from build123d import *

# Parameters (mm, degrees)
BOSS_EXTRUDE2_DEPTH         = 23
SHELL1_START                = 5
SHELL1_OUTLINE_W            = 16
SHELL1_OUTLINE_H            = 13
SHELL1_DEPTH                = 15
FILLET1_R                   = 2
FILLET3_R                   = 2
TAP_DRILL_FOR_M4X0_7_TAP1_D = 3.3


# Read off the part's stored shape, not the designer's step: Shell1
with BuildPart() as part:
    # Sketch1 → Boss-Extrude2 (new body)
    with BuildSketch(Plane.XY):
        Polygon((0, 0), (0, 20), (5, 20), (20, 5), (20, 0), align=None)
    extrude(amount=-BOSS_EXTRUDE2_DEPTH)

    # Shell1 outline → Shell1 (cut)
    with BuildSketch(Plane(origin=(0, 0, 0), x_dir=(1, 0, 0), z_dir=(0, 1, 0)).offset(SHELL1_START)):
        with Locations((13, 11.5)):
            Rectangle(SHELL1_OUTLINE_W, SHELL1_OUTLINE_H)
    extrude(amount=SHELL1_DEPTH, mode=Mode.SUBTRACT)

    # Fillet1
    fillet1_edges = [part.edges().sort_by_distance(p)[0] for p in [
        (12.5, 5, -18),
        (5, 12.5, -18),
        (5, 5, -11.5),
        (12.5, 5, -5),
        (5, 12.5, -5),
    ]]
    fillet(fillet1_edges, radius=FILLET1_R)

    # Fillet3
    fillet3_edges = [part.edges().sort_by_distance(p)[0] for p in [
        (2.5, 20, -23),
        (2.5, 20, 0),
        (20, 2.5, 0),
        (20, 2.5, -23),
        (0, 20, -11.5),
        (20, 0, -11.5),
    ]]
    fillet(fillet3_edges, radius=FILLET3_R)

    # Tap Drill for M4x0.7 Tap1 (through all)
    with Locations(Plane(origin=(5, 12, -11.5), x_dir=(0, 0, 1), z_dir=(1, 0, 0))):
        with Locations((0, 0)):
            Hole(TAP_DRILL_FOR_M4X0_7_TAP1_D / 2)

    # Sketch9 → CSK for M4 Flat Head Machine Screw2 (revolve, cut)
    with BuildSketch(Plane(origin=(12, 5, -11.5), x_dir=(0, 0, 1), z_dir=(1, 0, 0))):
        Polygon((0, 0), (0, 5), (2.25, 5), (2.25, 2.45), (4.7, 0), align=None)
    revolve(axis=Axis((12, 11.35, -11.5), (0, -1, 0)), mode=Mode.SUBTRACT)


solid = part.part
Here's how the part is built. I have some questions about the finished solid (model axes, mm). A direction names the side the tool comes from. Round coordinates to 2 decimals unless told otherwise and drop trailing zeros. Order: outer loops, then holes, each group sorted by start corner. A loop starts at its lowest first (then second) coordinate and runs counter-clockwise, first axis right, second up. Notation, with made-up numbers: (41, 76) -> (86, 76) arc R17 cw to (86, 100) -> close; hole circle Ø11 at (26, 72.25). An arc over 180 degrees is marked (long way). Use CSV: the item, a comma, the result in double quotes.
1. I want a section at C-C on y = 12. List the corners of the cut face in (x, z) for me.
Recorded:
outline,"(0, -23) -> (13, -23) -> (13, -18) -> (7, -18) arc R2 cw to (5, -16) -> (5, -13.15) -> (0, -13.15) -> close; (0, -9.85) -> (5, -9.85) -> (5, -7) arc R2 cw to (7, -5) -> (13, -5) -> (13, 0) -> (0, 0) -> close"
2. I want a section at A-A on z = -11.5. List the corners of the cut face in (x, y) for me.
Recorded:
outline,"(0, 0) -> (9.75, 0) -> (9.75, 2.55) -> (7.3, 5) -> (7, 5) arc R2 cw to (5, 7) -> (5, 10.35) -> (0, 10.35) -> close; (0, 13.65) -> (5, 13.65) -> (5, 20) -> (2, 20) arc R2 ccw to (0, 18) -> close; (14.25, 0) -> (18, 0) arc R2 ccw to (20, 2) -> (20, 5) -> (16.7, 5) -> (14.25, 2.55) -> close"
3. I'm going to push flat-ended pins straight in: P1, Ø2, axis at x = 12.5, z = -13.5, coming from the +Y side; P2, Ø5, axis at x = 12, z = -11.5, coming from the -Y side; P3, Ø5.5, axis at x = 15.5, z = -13, coming from the +Y side; P4, Ø1.1, axis at x = 8, z = -12, coming from the +Y side. Where does each tip first touch, or does it pass through?
Recorded:
P1,"stops at y = 3.36"
P2,"stops at y = 0"
P3,"stops at y = 5"
P4,"stops at y = 4.88"
4. I want a section at D-D on z = -19. List the corners of the cut face in (x, y) for me.
Recorded:
outline,"(0, 0) -> (18, 0) arc R2 ccw to (20, 2) -> (20, 5) -> (5, 20) -> (2, 20) arc R2 ccw to (0, 18) -> close"
5. I want a section at B-B on x = 12. List the corners of the cut face in (y, z) for me, and give its area (3 significant figures).
Recorded:
outline,"(0, -23) -> (13, -23) -> (13, -18) -> (7, -18) arc R2 cw to (5, -16) -> (5, -16.2) -> (2.55, -13.75) -> (0, -13.75) -> close; (0, -9.25) -> (2.55, -9.25) -> (5, -6.8) -> (5, -7) arc R2 cw to (7, -5) -> (13, -5) -> (13, 0) -> (0, 0) -> close"
area,"168 mm2"
6. Which directions (+Z, -Z, +X, -X, +Y, -Y) give clear straight access to the entire face, cutting with the end or side of a thin tool? Please do faces 4 (the face through (5.57, 5.6, -11.56)), 5 (the face through (0.6, 19.43, -11.66)).
Recorded:
face 4,"+X, +Y"
face 5,"+Z, -Z, -X, +Y"
7. Thinking about a two-plate mould opening in Z: for faces 1 (the face through (3.5, 19.2, -22.6)), 2 (the face through (7.2, 5, -12.2)), 3 (the face through (12, 13, -20)), which applies, pulls with the +Z half, pulls with the -Z half, needs draft (parallel to the pull), parting line crosses it, or undercut?
Recorded:
face 1,"pulls with the -Z half"
face 2,"undercut"
face 3,"needs draft"
8. I need wall thicknesses on line 1 along Y through (x, z) = (2.2, -11.5); line 2 along Z through (x, y) = (12, 1.45); line 3 along X through (y, z) = (7.5, -12). Which ranges of each line are inside material? Lowest first, please.
Recorded:
line 1,"y = 0 to 10.35, 13.65 to 20"
line 2,"z = -23 to -13.75, -9.25 to 0"
line 3,"x = 0 to 5"
